Verification items for the finished model (mm, model axes). Round coordinates to 2 decimals unless told otherwise and drop trailing zeros. Write each loop counter-clockwise with the first axis right and the second up, starting at its lowest first coordinate (ties: lowest second). Pieces come first, ordered by that corner, then holes. Notation, with made-up numbers: (-27.5, 84) - (18.5, 84) arc R11 ccw to (18.5, 99) - close; hole circle Ø11 at (58, -12). An arc over 180 degrees is marked (long way). Answer as a JSON object with one key per item and string values.
```python
from build123d import *

# Parameters (mm, degrees)
SALIENTE_EXTRUIR1_DEPTH = 2.7


with BuildPart() as part:
    # Croquis1 → Saliente-Extruir1 (new body)
    with BuildSketch(Plane.YZ):
        with BuildLine():
            Line((-22.110629153, -6.418985628), (-19.260629153, -6.418985628))
            Line((-19.260629153, -6.418985628), (-19.260629153, 0.059451181))
            Line((-19.260629153, 0.059451181), (-2.849889186, 0.059451181))
            Line((-2.849889186, 0.059451181), (-2.849889186, -6.418985628))
            Line((-2.849889186, -6.418985628), (0.000110814, -6.418985628))
            Line((0.000110814, -6.418985628), (0.000110814, 0.059451181))
            Line((0.000110814, 0.059451181), (16.410672264, 0.059451181))
            Line((16.410672264, 0.059451181), (16.410672264, -6.418985628))
            Line((16.410672264, -6.418985628), (19.260672264, -6.418985628))
            Line((19.260672264, -6.418985628), (19.260672264, 0.059451181))
            Line((19.260672264, 0.059451181), (35.671322972, 0.059451181))
            Line((35.671322972, 0.059451181), (35.671322972, -6.418985628))
            Line((35.671322972, -6.418985628), (38.521322972, -6.418985628))
            Line((38.521322972, -6.418985628), (38.521322972, 0.059451181))
            Line((38.521322972, 0.059451181), (54.93197368, 0.059451181))
            Line((54.93197368, 0.059451181), (54.93197368, -6.418985628))
            Line((54.93197368, -6.418985628), (57.78197368, -6.418985628))
            Line((57.78197368, -6.418985628), (57.78197368, 0))
            Line((57.78197368, 0), (92.811977714, 0))
            Line((92.811977714, 0), (92.840089973, -1.785119122))
            add(Edge.make_bspline(
                [(92.840089973, -1.785119122), (92.447237265, -2.064666353), (91.562107852, -2.694545376), (89.213895552, -3.700289956), (84.249349165, -5.617278564), (76.749898692, -7.957987248), (69.681676617, -9.820364855), (65.065941011, -10.77280706), (63.481529507, -10.891366405), (62.824262201, -10.940548819)],
                knots=[0, 0, 0, 0, 0.045739515, 0.103060799, 0.241853729, 0.552585532, 0.849009834, 0.937364189, 1, 1, 1, 1], degree=3))
            Line((62.824262201, -10.940548819), (30.594296183, -10.940548819))
            add(Edge.make_bspline(
                [(30.594296183, -10.940548819), (30.921447359, -11.442137244), (31.555538234, -12.414367523), (31.268248789, -14.173159627), (30.182416548, -15.592511875), (29.034537635, -15.791382717), (28.440778339, -15.894254382)],
                knots=[0, 0, 0, 0, 0.257583929, 0.499275666, 0.740985929, 1, 1, 1, 1], degree=3))
            add(Edge.make_bspline(
                [(28.440778339, -15.894254382), (27.847016865, -15.79138162), (26.69915531, -15.59250767), (25.61335925, -14.173151066), (25.326077358, -12.414363927), (25.960178406, -11.442136771), (26.287321547, -10.940548819)],
                knots=[0, 0, 0, 0, 0.259010563, 0.500720038, 0.74241327, 1, 1, 1, 1], degree=3))
            Line((26.287321547, -10.940548819), (-59.95124774, -10.940548819))
            add(Edge.make_bspline(
                [(-59.95124774, -10.940548819), (-59.624096976, -11.442137347), (-58.990006223, -12.414367218), (-59.277284868, -14.1731508), (-60.363078616, -15.592503731), (-61.510934237, -15.79138053), (-62.104659968, -15.894254382)],
                knots=[0, 0, 0, 0, 0.257586595, 0.499280522, 0.740990692, 1, 1, 1, 1], degree=3))
            add(Edge.make_bspline(
                [(-62.104659968, -15.894254382), (-62.737656591, -15.777608826), (-63.958163548, -15.552699707), (-65.026875083, -13.971822996), (-65.172920695, -12.072708959), (-64.363662916, -11.135174473), (-63.944611922, -10.649752914)],
                knots=[0, 0, 0, 0, 0.259500482, 0.500353607, 0.74130111, 1, 1, 1, 1], degree=3))
            add(Edge.make_bspline(
                [(-63.944611922, -10.649752914), (-65.124297825, -10.468220396), (-67.923268081, -10.037509037), (-72.470849105, -9.093983121), (-78.212469404, -7.520495573), (-83.096036068, -5.527641263), (-86.600780666, -2.667344706), (-87.002807809, -0.84127357), (-87.188022286, 0)],
                knots=[0, 0, 0, 0, 0.133262352, 0.316183621, 0.518474271, 0.796547325, 0.906269063, 1, 1, 1, 1], degree=3))
            Line((-87.188022286, 0), (-60.631930569, 0))
            Line((-60.631930569, 0), (-60.631930569, -6.478436809))
            Line((-60.631930569, -6.478436809), (-57.781930569, -6.478436809))
            Line((-57.781930569, -6.478436809), (-57.781930569, 0.059451181))
            Line((-57.781930569, 0.059451181), (-41.371279861, 0.059451181))
            Line((-41.371279861, 0.059451181), (-41.371279861, -6.418985628))
            Line((-41.371279861, -6.418985628), (-38.521279861, -6.418985628))
            Line((-38.521279861, -6.418985628), (-38.521279861, 0.059451181))
            Line((-38.521279861, 0.059451181), (-22.110629153, 0.059451181))
            Line((-22.110629153, 0.059451181), (-22.110629153, -6.418985628))
        make_face()
    extrude(amount=SALIENTE_EXTRUIR1_DEPTH)


solid = part.part
```
1. Material ranges on probe 1 along Z at (x, y) = (0.9, 10); probe 2 along Z at (x, y) = (0.9, -2.5); probe 3 along Y at (x, z) = (2.65, -14), recorded low to high. Write a range as from..to.
Completed:
{"probe 1": "z = -10.94..0.06", "probe 2": "z = -10.94..-6.42", "probe 3": "y = -64.85..-59.36, 25.7..31.19"}
2. Cross-section at B-B (z = -4.5). Count the separate pieces of the cut face and the enclosed holes in it, plus the area to 3 significant figures.
Completed:
{"separate pieces": "8", "enclosed holes": "0", "area": "409 mm^2"}
3. Mould release check, pull along X, two halves, no side actions. Record for faces 1 (the face through (0, 4, -4)), 2 (the face through (2.7, 4, -4)): released by +X, released by -X, zero draft, split by the parting line, or undercut.
Completed:
{"face 1": "released by -X", "face 2": "released by +X"}
4. Go/stop test with flat-tipped pins: pin 1 (0.8 mm diameter, centred on x = 1.5, y = 17.5, fed in from +Z); pin 2 (1.4 mm diameter, centred on x = 1.5, z = -3.5, fed in from -Y); pin 3 (0.8 mm diameter, centred on x = 1.5, z = -4, fed in from -Y). Record where each tip stops, or that it passes through.
Completed:
{"pin 1": "stops at z = -6.42", "pin 2": "stops at y = -86.13", "pin 3": "stops at y = -85.39"}
5. Cross-section at A-A (y = -51.5). Record the boundary of the cut face in (x, z).
Completed:
{"outline": "(0, -10.94) - (2.7, -10.94) - (2.7, 0.06) - (0, 0.06) - close"}
